Read the model definition and answer for the solid it produces. Units are mm, in the model's axes. Face numbers are marked on the shaded views. A direction names the side the tool comes from. Coordinates: 2 decimals unless noted, no trailing zeros. Loops run counter-clockwise (first coordinate to the right, second up) from the corner with the lowest first, then second, coordinate; pieces in that order, holes last. Notation, with made-up numbers: M 68.25,66 L 76.25,66 A24 ccw 76.25,104 Z; hole C 38,30.5 d7. An arc over 180 degrees is marked long. One line per item, written item: value. Start each with the question number.
1. The part is cut by section A-A (z = -1). Write down the section's boundary in (x, y), then the cut area to 3 significant figures.
2. Consider probe 1 along Y at (x, z) = (18, 0.2); probe 2 along Y at (x, z) = (16.5, -1.4); probe 3 along Y at (x, z) = (18, -1.3). Determine where each line is inside the solid, lowest interval first.
3. The part is cut by section D-D (z = 1.2). Write down the section's boundary in (x, y).
4. Determine the mould class of the marked faces 1, 2, 3 and 4 for opening direction Z: +Z half, -Z half, draft (parallel to the pull), parting line (faces both ways), or undercut.
5. The part is cut by section B-B (x = 18). Write down the section's boundary in (y, z).
6. The part is cut by section C-C (y = -4.5). Write down the section's boundary in (x, z), then the cut area to 3 significant figures.
7. For the marked faces 5, 6 and 7, determine the directions among +Z, -Z, +X, -X, +Y, -Y from which every point of the face is accessible in a straight line to the end or side of a thin tool.
8. Flat-ended cylindrical pins translate along their axes: pin 1 (1.7 mm diameter, centred on x = 12, y = 0, fed in from -Z); pin 2 (0.6 mm diameter, centred on x = 18, z = -1.5, fed in from -Y); pin 3 (1.2 mm diameter, centred on x = 12, y = -0.5, fed in from +Z). Find the tip coordinate at first contact, or state that the pin passes through.
```python
from build123d import *

# Parameters (mm, degrees)
BOSS_EXTRUDE1_DEPTH = 2
BOSS_EXTRUDE2_START = 2.5
BOSS_EXTRUDE2_DEPTH = 2.5
CUT_EXTRUDE1_DEPTH  = 2.5
BOSS_EXTRUDE3_DEPTH = 2.3
SKETCH9_R           = 2.1
CUT_EXTRUDE2_DEPTH  = 2.5
SKETCH10_R          = 2.5
BOSS_EXTRUDE4_DEPTH = 1.2
SKETCH11_R          = 0.95
CUT_EXTRUDE3_DEPTH  = 9.2
SKETCH12_R          = 2
CUT_EXTRUDE4_DEPTH  = 2.5
SKETCH14_W          = 20.343145751
SKETCH14_H          = 1.841510486
SKETCH14_W_2        = 17
SKETCH14_H_2        = 1.34163614
BOSS_EXTRUDE5_DEPTH = 1.2
FILLET1_R           = 1.5
SKETCH17_R          = 0.95
CUT_EXTRUDE5_DEPTH  = 3


# Read off the part's stored shape, not the designer's step: Boss-Extrude3
with BuildPart() as part:
    # Sketch5 → Boss-Extrude1 (new body)
    with BuildSketch(Plane.XY):
        with BuildLine():
            Line((8, 0), (9, -2.501635265))
            Line((9, -2.501635265), (9, -7.001635265))
            Line((9, -7.001635265), (26, -7.001635265))
            Line((26, -7.001635265), (26, 7.498364735))
            Line((26, 7.498364735), (5.656854249, 7.498364735))
            Line((5.656854249, 7.498364735), (5.656854249, 5.656854249))
            ThreePointArc((5.656854249, 5.656854249), (7.39103626, 3.061467459), (8, 0))
        make_face()
    extrude(amount=BOSS_EXTRUDE1_DEPTH)

    # Sketch6 → Boss-Extrude2 (add)
    with BuildSketch(Plane(origin=(0, 0, 0), x_dir=(-1, 0, 0), z_dir=(0, 0, -1)).offset(BOSS_EXTRUDE2_START)):
        with BuildLine():
            Line((-5.656854249, 7.498364735), (-5.656854249, 5.656854249))
            ThreePointArc((-5.656854249, 5.656854249), (-7.39103626, 3.061467459), (-8, 0))
            Line((-8, 0), (-9, -2.501635265))
            Line((-9, -2.501635265), (-9, -7.001635265))
            Line((-9, -7.001635265), (-26, -7.001635265))
            Line((-26, -7.001635265), (-26, 7.498364735))
            Line((-26, 7.498364735), (-5.656854249, 7.498364735))
        make_face()
    extrude(amount=-BOSS_EXTRUDE2_DEPTH)

    # Sketch7 → Cut-Extrude1 (cut)
    with BuildSketch(Plane(origin=(0, 0, -2.5), x_dir=(-1, 0, 0), z_dir=(0, 0, -1))):
        Polygon((-26, 5.298364735), (-2.738141148, 5.298364735), (-2.738141148, 3.998364735), (-29.849535112, 3.998364735), (-29.849535112, 5.298364735), align=None)
    extrude(amount=-CUT_EXTRUDE1_DEPTH, mode=Mode.SUBTRACT)

    # Boss-Extrude3 outline → Boss-Extrude3 (add)
    with BuildSketch(Plane(origin=(0, 0, -2.5), x_dir=(-1, 0, 0), z_dir=(0, 0, -1))):
        with BuildLine():
            Line((-9, -7.001635265), (-9, -5.659999125))
            Line((-9, -5.659999125), (0, -5.659998688))
            ThreePointArc((0, -5.659998688), (5.659998688, 0), (0, 5.659998688))
            Line((0, 5.659998688), (-5.656854249, 5.656854249))
            Line((-5.656854249, 5.656854249), (-5.656854249, 7.498364735))
            Line((-5.656854249, 7.498364735), (-26, 7.498364735))
            Line((-26, 7.498364735), (-26, -7.001635265))
            Line((-26, -7.001635265), (-9, -7.001635265))
        make_face()
    extrude(amount=BOSS_EXTRUDE3_DEPTH)

    # Sketch9 → Cut-Extrude2 (cut)
    with BuildSketch(Plane(origin=(0, 0, -4.8), x_dir=(-1, 0, 0), z_dir=(0, 0, -1))):
        Circle(SKETCH9_R)
    extrude(amount=-CUT_EXTRUDE2_DEPTH, mode=Mode.SUBTRACT)

    # Sketch10 → Boss-Extrude4 (add)
    with BuildSketch(Plane(origin=(0, 0, -4.8), x_dir=(-1, 0, 0), z_dir=(0, 0, -1))):
        with Locations((-12, 0)):
            Circle(SKETCH10_R)
        with Locations((-18, 0)):
            Circle(SKETCH10_R)
    extrude(amount=BOSS_EXTRUDE4_DEPTH)

    # Sketch11 → Cut-Extrude3 (cut)
    with BuildSketch(Plane(origin=(0, 0, -6), x_dir=(-1, 0, 0), z_dir=(0, 0, -1))):
        with Locations((-18, 0)):
            Circle(SKETCH11_R)
        with Locations((-12, 0)):
            Circle(SKETCH11_R)
    extrude(amount=-CUT_EXTRUDE3_DEPTH, mode=Mode.SUBTRACT)

    # Sketch12 → Cut-Extrude4 (cut)
    with BuildSketch(Plane.XY.offset(2)):
        with Locations((12, 0)):
            Circle(SKETCH12_R)
        with Locations((18, 0)):
            Circle(SKETCH12_R)
    extrude(amount=-CUT_EXTRUDE4_DEPTH, mode=Mode.SUBTRACT)

    # Sketch14 → Boss-Extrude5 (add)
    with BuildSketch(Plane(origin=(0, 0, -4.8), x_dir=(-1, 0, 0), z_dir=(0, 0, -1))):
        with Locations((-15.828427124, 6.577609492)):
            Rectangle(SKETCH14_W, SKETCH14_H)
        with Locations((-17.5, -6.330817195)):
            Rectangle(SKETCH14_W_2, SKETCH14_H_2)
    extrude(amount=BOSS_EXTRUDE5_DEPTH)

    # Fillet1
    # the kernel refuses this fillet: 1.5 mm, written as the material it takes off along each edge
    with BuildSketch(Plane(origin=(24.5, -5.501635265, 0.5), x_dir=(0, 0, 1), z_dir=(0, -1, 0))) as fillet1_piece_1_section:
        Polygon((0, 0), (FILLET1_R, 0), (FILLET1_R, -FILLET1_R), (0, -FILLET1_R), align=None)
    fillet1_piece_1 = extrude(amount=FILLET1_R, mode=Mode.PRIVATE)
    fillet1_piece_1 = fillet1_piece_1 - Plane(origin=(24.5, -5.501635265, 0.5), x_dir=(-0.7071067811865475, 0, -0.7071067811865475), z_dir=(0, -1, 0)) * Sphere(FILLET1_R, mode=Mode.PRIVATE)
    add(fillet1_piece_1, mode=Mode.SUBTRACT)
    with BuildSketch(Plane(origin=(24.5, 5.998364735, 0.5), x_dir=(0, 0, 1), z_dir=(0, 1, 0))) as fillet1_piece_2_section:
        Polygon((0, 0), (FILLET1_R, 0), (FILLET1_R, FILLET1_R), (0, FILLET1_R), align=None)
    fillet1_piece_2 = extrude(amount=FILLET1_R, mode=Mode.PRIVATE)
    fillet1_piece_2 = fillet1_piece_2 - Plane(origin=(24.5, 5.998364735, 0.5), x_dir=(-0.7071067811865475, 0, -0.7071067811865475), z_dir=(0, 1, 0)) * Sphere(FILLET1_R, mode=Mode.PRIVATE)
    add(fillet1_piece_2, mode=Mode.SUBTRACT)
    with BuildSketch(Plane(origin=(26, -5.501635265, 2), x_dir=(-1, 0, 0), z_dir=(0, 1, 0))) as fillet1_piece_3:
        with BuildLine():
            CenterArc((FILLET1_R, -FILLET1_R), FILLET1_R, 90, 90)
            Line((0, -FILLET1_R), (0, 0))
            Line((0, 0), (FILLET1_R, 0))
        make_face()
    extrude(amount=11.5, mode=Mode.SUBTRACT)
    with BuildSketch(Plane(origin=(26, -7.001635265, -2.5), x_dir=(-1, 0, 0), z_dir=(0, 0, 1))) as fillet1_piece_4:
        with BuildLine():
            CenterArc((FILLET1_R, -FILLET1_R), FILLET1_R, 90, 90)
            Line((0, -FILLET1_R), (0, 0))
            Line((0, 0), (FILLET1_R, 0))
        make_face()
    extrude(amount=3, mode=Mode.SUBTRACT)
    with BuildSketch(Plane(origin=(5.25, -7.001635265, 2), x_dir=(0, 1, 0), z_dir=(1, 0, 0))) as fillet1_piece_5:
        with BuildLine():
            CenterArc((FILLET1_R, -FILLET1_R), FILLET1_R, 90, 90)
            Line((0, -FILLET1_R), (0, 0))
            Line((0, 0), (FILLET1_R, 0))
        make_face()
    extrude(amount=19.25, mode=Mode.SUBTRACT)
    with BuildSketch(Plane(origin=(24.5, 7.498364735, 2), x_dir=(0, -1, 0), z_dir=(-1, 0, 0))) as fillet1_piece_6:
        with BuildLine():
            CenterArc((FILLET1_R, -FILLET1_R), FILLET1_R, 90, 90)
            Line((0, -FILLET1_R), (0, 0))
            Line((0, 0), (FILLET1_R, 0))
        make_face()
    extrude(amount=22.593145751, mode=Mode.SUBTRACT)
    with BuildSketch(Plane(origin=(26, 7.498364735, -2.5), x_dir=(-1, 0, 0), z_dir=(0, 0, 1))) as fillet1_piece_7:
        with BuildLine():
            CenterArc((FILLET1_R, FILLET1_R), FILLET1_R, 180, 90)
            Line((0, FILLET1_R), (0, 0))
            Line((0, 0), (FILLET1_R, 0))
        make_face()
    extrude(amount=3, mode=Mode.SUBTRACT)
    with BuildSketch(Plane(origin=(26, 7.498364735, -2.5), x_dir=(-1.0, -1.9174232572065026e-10, 0), z_dir=(0, 0, -1))) as fillet1_piece_8:
        with BuildLine():
            CenterArc((FILLET1_R, -FILLET1_R), FILLET1_R, 90.000000011, 90)
            Line((FILLET1_R * 1.9173522033e-10, -FILLET1_R), (0, 0))
            Line((0, 0), (FILLET1_R, 0))
        make_face()
    extrude(amount=2.3, mode=Mode.SUBTRACT)
    with BuildSketch(Plane(origin=(26, 7.498364735, -4.8), x_dir=(-1, 0, 0), z_dir=(0, 0, -1))) as fillet1_piece_9:
        with BuildLine():
            CenterArc((FILLET1_R, -FILLET1_R), FILLET1_R, 90, 90)
            Line((0, -FILLET1_R), (0, 0))
            Line((0, 0), (FILLET1_R, 0))
        make_face()
    extrude(amount=4.95, mode=Mode.SUBTRACT)
    with BuildSketch(Plane(origin=(26, -7.001635265, -2.5), x_dir=(-1.0, -1.9169850891861218e-10, 0), z_dir=(0, 0, -1))) as fillet1_piece_10:
        with BuildLine():
            CenterArc((FILLET1_R, FILLET1_R), FILLET1_R, 180.000000011, 90)
            Line((-FILLET1_R * 1.91707982785e-10, FILLET1_R), (0, 0))
            Line((0, 0), (FILLET1_R, 0))
        make_face()
    extrude(amount=2.3, mode=Mode.SUBTRACT)
    with BuildSketch(Plane(origin=(26, -7.001635265, -4.8), x_dir=(-1, 0, 0), z_dir=(0, 0, -1))) as fillet1_piece_11:
        with BuildLine():
            CenterArc((FILLET1_R, FILLET1_R), FILLET1_R, 180, 90)
            Line((0, FILLET1_R), (0, 0))
            Line((0, 0), (FILLET1_R, 0))
        make_face()
    extrude(amount=4.95, mode=Mode.SUBTRACT)

    # Sketch17 → Cut-Extrude5 (cut)
    with BuildSketch(Plane.XZ.offset(7.001635265)):
        with Locations((22, -1)):
            Circle(SKETCH17_R)
        with Locations((18, -1)):
            Circle(SKETCH17_R)
    extrude(amount=-CUT_EXTRUDE5_DEPTH, mode=Mode.SUBTRACT)


with BuildPart() as body_2:
    # Split1: the piece on the far side of the plane
    add(part.part)
    split(bisect_by=Plane(origin=(0, 0, -2.5), x_dir=(-1, 0, 0), z_dir=(0, 0, -1)), keep=Keep.BOTTOM)


with BuildPart() as part_1:
    add(part.part)

    # Split1
    split(bisect_by=Plane(origin=(0, 0, -2.5), x_dir=(-1, 0, 0), z_dir=(0, 0, -1)), keep=Keep.TOP)


solid = body_2.part
```
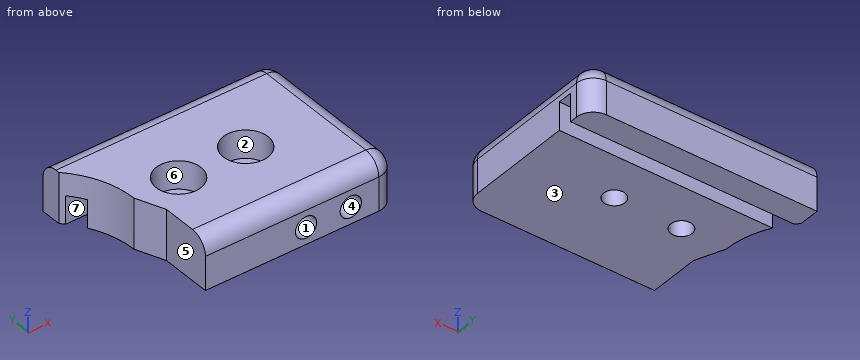
Answer block:
1. outline: M 5.66,5.66 A8 cw 5.99,5.3 L 26,5.3 L 26,6 A1.5 ccw 24.5,7.5 L 5.66,7.5 Z; M 6.93,4 A8 cw 8,0 L 9,-2.5 L 9,-7 L 17.05,-7 L 17.05,-4 L 18.95,-4 L 18.95,-7 L 21.05,-7 L 21.05,-4 L 22.95,-4 L 22.95,-7 L 24.5,-7 A1.5 ccw 26,-5.5 L 26,4 Z; hole C 12,0 d1.9; hole C 18,0 d1.9
1. area: 220 mm2
2. probe 1: y = -7 to -2, 2 to 7.5
2. probe 2: y = -7 to 4, 5.3 to 7.5
2. probe 3: y = -4 to -0.95, 0.95 to 4, 5.3 to 7.5
3. outline: M 5.66,5.66 A8 cw 8,0 L 9,-2.5 L 9,-6.83 L 24.5,-6.83 A1.33 ccw 25.83,-5.5 L 25.83,6 A1.33 ccw 24.5,7.33 L 5.66,7.33 Z; hole C 12,0 d4; hole C 18,0 d4
4. face 1: undercut
4. face 2: draft
4. face 3: -Z half
4. face 4: undercut
5. outline: M -7,-2.5 L -0.95,-2.5 L -0.95,-0.5 L -2,-0.5 L -2,2 L -5.5,2 A1.5 ccw -7,0.5 L -7,-0.05 L -4,-0.05 L -4,-1.95 L -7,-1.95 Z; M 0.95,-2.5 L 4,-2.5 L 4,0 L 5.3,0 L 5.3,-2.5 L 7.5,-2.5 L 7.5,0.5 A1.5 ccw 6,2 L 2,2 L 2,-0.5 L 0.95,-0.5 Z
6. outline: M 9,-2.5 L 26,-2.5 L 26,0.5 A1.5 ccw 24.5,2 L 9,2 Z; hole C 18,-1 d1.9; hole C 22,-1 d1.9
6. area: 70.3 mm2
7. face 5: +Z, -Z, -X, -Y
7. face 6: +Z
7. face 7: -Z, +X, -X
8. pin 1: passes through
8. pin 2: stops at y = -4
8. pin 3: stops at z = -0.5
